The listing builds one solid part. Answer for the finished solid, in the listing's coordinates (mm). A direction names the side the tool comes from. Round coordinates to 2 decimals unless told otherwise and drop trailing zeros. Loops run counter-clockwise (first coordinate to the right, second up) from the corner with the lowest first, then second, coordinate; pieces in that order, holes last. Notation, with made-up numbers: (12, 70) - (49, 70) arc R22 cw to (49, 106) - close; hole circle Ø4 at (69.25, -1). An arc over 180 degrees is marked (long way). Write item = value, one per line. Start each with the question number.
1) A tool of negligible diameter and unlimited length cuts with its end or side. For faces 1 (the flat face through (3, 16, 444)), 2 (the flat face through (0, 16, 444)), 3 (the flat face through (0, 0, 444)), from which of +Z, -Z, +X, -X, +Y, -Y can it reach the whole face along a straight path? Write none if from no direction.
2) Section A-A, the plane z = 841.5 is taken. Determine the outline of the cut face in (x, y), and give its area (3 significant figures).
3) Given pin 1 Ø6 at (y, z) = (18, 435) entering from -X; pin 2 Ø4 at (y, z) = (16, 668.5) entering from +X; pin 3 Ø6 at (x, z) = (-15, 885) entering from +Y; pin 4 Ø2.5 at (x, z) = (18, 885) entering from -Y, each flat-ended and moving along its own axis, determine where each tip first touches the part or whether it passes through.
4) Straight lines are drawn through the part: line 1 along X through (y, z) = (2.1, 885) (3 decimals); line 2 along Z through (x, y) = (1, 18) (3 decimals); line 3 along X through (y, z) = (8.5, 236.5). For each, find the intervals that lie inside material, in ascending order.
Autodesk Inventor part; units mm, degrees
ref_plane "YZ Plane" through (0, 0, 0) normal (1, 0, 0) x (0, 1, 0)
ref_plane "XZ Plane" through (0, 0, 0) normal (0, 1, 0) x (-1, 0, 0)
ref_plane "XY Plane" through (0, 0, 0) normal (0, 0, 1) x (1, 0, 0)
sketch "Sketch1" plane through (0, 0, 0) normal (0, 0, 1) x (1, 0, 0)
  line L0 (0, 0) -> (30, 0)
  line L1 (30, 0) -> (30, 3)
  line L2 (30, 3) -> (3, 3)
  line L3 (3, 3) -> (3, 30)
  line L4 (3, 30) -> (0, 30)
  line L5 (0, 0) -> (-30, 0)
  line L6 (-30, 0) -> (-30, 3)
  line L7 (-30, 3) -> (0, 3)
  line L8 (0, 3) -> (0, 30)
  dimension "d0" = 3
  dimension "d2" = 30
  dimension "d5" = 3
extrude "Extrusion1" add sketch "Sketch1" along normal blind 900
sketch "Sketch2" plane through (3, 3, 900) normal (0, 1, 0) x (1, 0, 0)
  line L0 (-3, 0) -> (-33, 0)
  line L1 (-3, 900) -> (-3, 0)
  line L2 (0, 900) -> (0, 0)
  line L3 (27, 0) -> (0, 0)
  point P0 (15, 15)
  point P1 (-18, 15)
  point P2 (-18, 465)
  point P3 (15, 465)
  point P4 (15, 915)
  point P5 (-18, 915)
  point P6 (-18, 1365)
  point P7 (15, 1365)
  dimension "d8" = 15
  dimension "d9" = 15
  dimension "d10" = 15
  dimension "d11" = 15
  dimension "d12" = 450
  dimension "d13" = 450
  dimension "d14" = 15
  dimension "d15" = 15
  dimension "d16" = 450
  dimension "d17" = 450
  dimension "d18" = 15
  dimension "d19" = 15
  dimension "d20" = 450
  dimension "d21" = 450
  dimension "d22" = 15
  dimension "d23" = 15
hole "Hole1" at (18, 3, 885) at (-15, 3, 885) at (-15, 3, 435) at (18, 3, 435) at (18, 3, -15) at (-15, 3, -15) at (-15, 3, -465) at (18, 3, -465) direction (0, -1, 0) diameter 3.81 end through all
sketch "Sketch3" plane through (3, 30, 900) normal (1, 0, 0) x (0, 0, -1)
  line L0 (0, -27) -> (0, 0)
  line L1 (900, -27) -> (0, -27)
  point P0 (900, -30)
  point P1 (15, -12)
  point P2 (465, -12)
  point P3 (915, -12)
  point P4 (1365, -12)
  dimension "d31" = 15
  dimension "d32" = 15
  dimension "d33" = 450
  dimension "d34" = 15
  dimension "d35" = 450
  dimension "d36" = 450
  dimension "d37" = 15
  dimension "d38" = 15
hole "Hole2" at (3, 18, 885) at (3, 18, 435) at (3, 18, -15) at (3, 18, -465) direction (-1, 0, 0) diameter 3.81 end through all
equation "\"d0\" = Thickness"
equation "\"d2\" = Width"
equation "\"d5\" = Thickness"
equation "\"d6\" = Height"
equation "\"Width\" = 30"
equation "\"Thickness\" = 3"
equation "\"Height\" = 900"
equation "\"HoleDistance\" = 15"
properties part number "mid90"
Geometry check:
q1.face_1 = +Z, -Z, +X, +Y
q1.face_2 = +Z, -Z, -X, +Y
q1.face_3 = +Z, -Z, +X, -X, -Y
q2.outline = (-30, 0) - (30, 0) - (30, 3) - (3, 3) - (3, 30) - (0, 30) - (0, 3) - (-30, 3) - close
q2.area = 261 mm2
q3.pin_1 = 0
q3.pin_2 = 3
q3.pin_3 = 3
q3.pin_4 = through
q4.line_1 = -30 to -16.905, -13.095 to 16.095, 19.905 to 30
q4.line_2 = 0 to 433.095, 436.905 to 883.095, 886.905 to 900
q4.line_3 = 0 to 3
